```python
from build123d import *

# Parameters (mm, degrees)
SKETCH1_W           = 101.6
SKETCH1_H           = 50.8
BOSS_EXTRUDE1_DEPTH = 25.4
SKETCH2_W           = 76.2
SKETCH2_H           = 19.05
BOSS_EXTRUDE2_DEPTH = 50.8
CUT_EXTRUDE1_DEPTH  = 26.4
SKETCH4_R           = 3.175
CUT_EXTRUDE3_DEPTH  = 26.4
SKETCH4_3_R         = 9.525
SKETCH4_3_R_2       = 3.175
BOSS_EXTRUDE3_DEPTH = 3.175
SKETCH5_R           = 6.35
CUT_EXTRUDE4_DEPTH  = 26.4


with BuildPart() as part:
    # Sketch1 → Boss-Extrude1 (new body)
    with BuildSketch(Plane(origin=(0, 0, 0), x_dir=(1, 0, 0), z_dir=(0, 1, 0))):
        with Locations((50.8, 25.4)):
            Rectangle(SKETCH1_W, SKETCH1_H)
    extrude(amount=BOSS_EXTRUDE1_DEPTH)

    # Sketch2 → Boss-Extrude2 (add)
    with BuildSketch(Plane(origin=(0, 25.4, 0), x_dir=(1, 0, 0), z_dir=(0, 1, 0))):
        with Locations((57.15, 34.925)):
            Rectangle(SKETCH2_W, SKETCH2_H)
    extrude(amount=BOSS_EXTRUDE2_DEPTH)

    # Sketch3 → Cut-Extrude1 (cut, through all)
    with BuildSketch(Plane.XY.offset(-25.4)):
        Polygon((19.05, 76.2), (95.25, 76.2), (19.05, 25.4), align=None)
    extrude(amount=-CUT_EXTRUDE1_DEPTH, mode=Mode.SUBTRACT)

    # Sketch4 → Cut-Extrude3 (cut, through all)
    with BuildSketch(Plane.XY.offset(-25.4)):
        with Locations((84.791572172, 56.416317707)):
            Circle(SKETCH4_R)
    extrude(amount=-CUT_EXTRUDE3_DEPTH, mode=Mode.SUBTRACT)

    # Sketch4_3 → Boss-Extrude3 (add)
    with BuildSketch(Plane.XY.offset(-25.4)):
        with Locations(Location((84.791572172, 56.416317707, 0), (0, 0, 180))):  # turned: the seam where the file's is
            Circle(SKETCH4_3_R)
        with Locations((84.791572172, 56.416317707)):
            Circle(SKETCH4_3_R_2, mode=Mode.SUBTRACT)
    extrude(amount=BOSS_EXTRUDE3_DEPTH)

    # Sketch5 → Cut-Extrude4 (cut, through all)
    with BuildSketch(Plane(origin=(0, 25.4, 0), x_dir=(1, 0, 0), z_dir=(0, 1, 0))):
        with Locations(Location((19.05, 12.7, 0), (0, 0, 270))):  # turned: the seam where the file's is
            Circle(SKETCH5_R)
        with Locations(Location((82.55, 12.7, 0), (0, 0, 270))):  # turned: the seam where the file's is
            Circle(SKETCH5_R)
    extrude(amount=-CUT_EXTRUDE4_DEPTH, mode=Mode.SUBTRACT)


solid = part.part
```
Source: CAD feature listing. Evaluate the final solid. Frame: model axes, mm. A direction names the side the tool comes from. Round coordinates to 2 decimals unless told otherwise and drop trailing zeros. Loops run counter-clockwise (first coordinate to the right, second up) from the corner with the lowest first, then second, coordinate; pieces in that order, holes last.
1. Ray query, L1, parallel to X at y = 6, z = -10; L2, parallel to Z at x = 82, y = 19; L3, parallel to X at y = 23.5, z = -13.5. Return the intervals inside material, ascending.
2. Mould query, pull axis Y, two halves, no side actions, for faces 5 (the flat face through (65, 39, -25.4)), 6 (the flat face through (50, 0, -26)), 7 (the cylindrical face through (75.99, 60.06, -23.83)), 8 (the flat face through (101.6, 13, -25)). Classes: released by +Y, released by -Y, zero draft, split by the parting line, or undercut.
3. Section query C-C on x = 53.5. Output: boundary loops of the cut face in (y, z), and give its area (3 significant figures).
4. Section query A-A on z = -12.7. Output: boundary loops of the cut face in (x, y), and give its area (3 significant figures).
5. Contact query for flat-ended pins moving along their axis: pin 1 (4 mm diameter, centred on x = 84.79, y = 56.42, fed in from -Z); pin 2 (21 mm diameter, centred on x = 86, y = 53, fed in from +Z) (3 decimals); pin 3 (4 mm diameter, centred on x = 36.5, y = 38.5, fed in from +Z); pin 4 (21 mm diameter, centred on y = 55.5, z = -31.5, fed in from +X). Output: stop coordinate, or through.
6. Section query B-B on x = 16.5. Output: boundary loops of the cut face in (y, z), and give its area (3 significant figures).
7. Section query D-D on y = 39.5. Output: boundary loops of the cut face in (x, z), and give its area (3 significant figures).
8. Access query for faces 1 (the flat face through (50, 13, 0)), 2 (the flat face through (81, 56, -22.225)), 3 (the flat face through (74, 39, -44.45)), 4 (the flat face through (95.25, 50, -35)). Directions: +Z, -Z, +X, -X, +Y, -Y. A direction counts if a zero-diameter tool reaches every point of the face in a straight line with its end or side. Return the directions, or none.
Answers below:
1. L1: x = 0 to 13.3, 24.8 to 76.8, 88.3 to 101.6
1. L2: z = -50.8 to -19.03, -6.37 to 0
1. L3: x = 0 to 12.75, 25.35 to 76.25, 88.85 to 101.6
2. face 5: undercut
2. face 6: released by -Y
2. face 7: undercut
2. face 8: zero draft
3. outline: (0, -50.8) - (25.4, -50.8) - (25.4, -44.45) - (48.37, -44.45) - (48.37, -25.4) - (25.4, -25.4) - (25.4, 0) - (0, 0) - close
3. area: 1,730 mm2
4. outline: (0, 0) - (12.7, 0) - (12.7, 25.4) - (0, 25.4) - close; (25.4, 0) - (76.2, 0) - (76.2, 25.4) - (25.4, 25.4) - close; (88.9, 0) - (101.6, 0) - (101.6, 25.4) - (88.9, 25.4) - close
4. area: 1,940 mm2
5. pin 1: passes through
5. pin 2: stops at z = -22.225
5. pin 3: stops at z = -25.4
5. pin 4: stops at x = 95.25
6. outline: (0, -50.8) - (25.4, -50.8) - (25.4, -18.52) - (0, -18.52) - close; (0, -6.88) - (25.4, -6.88) - (25.4, 0) - (0, 0) - close
6. area: 995 mm2
7. outline: (40.2, -44.45) - (95.25, -44.45) - (95.25, -25.4) - (40.2, -25.4) - close
7. area: 1,050 mm2
8. face 1: +Z, +X, -X, +Y, -Y
8. face 2: +Z, +X, -X, +Y
8. face 3: -Z, +X, -X, +Y
8. face 4: +Z, -Z, +X, +Y
